from build123d import *

# Parameters (mm, degrees)
SKETCH1_W           = 17.4
SKETCH1_H           = 16.3
BOSS_EXTRUDE1_DEPTH = 5.6
SKETCH2_R           = 4.25
BOSS_EXTRUDE2_DEPTH = 7
SKETCH3_R           = 2.9
BOSS_EXTRUDE3_DEPTH = 13
FILLET1_R           = 3
SKETCH4_W           = 3.8
SKETCH4_H           = 0.8
BOSS_EXTRUDE4_DEPTH = 2.9
FILLET2_R           = 1
BOSS_EXTRUDE5_DEPTH = 2.3


with BuildPart() as part:
    # Sketch1 → Boss-Extrude1 (new body)
    with BuildSketch(Plane(origin=(0, 0, 0), x_dir=(1, 0, 0), z_dir=(0, 1, 0))):
        Rectangle(SKETCH1_W, SKETCH1_H)
    extrude(amount=BOSS_EXTRUDE1_DEPTH)

    # Sketch2 → Boss-Extrude2 (add)
    with BuildSketch(Plane(origin=(0, 5.6, 0), x_dir=(1, 0, 0), z_dir=(0, 1, 0))):
        with Locations(Location((0, 0, 0), (0, 0, 270))):  # turned: the seam where the file's is
            Circle(SKETCH2_R)
    extrude(amount=BOSS_EXTRUDE2_DEPTH)

    # Sketch3 → Boss-Extrude3 (add)
    with BuildSketch(Plane(origin=(0, 12.6, 0), x_dir=(1, 0, 0), z_dir=(0, 1, 0))):
        with Locations(Location((0, 0, 0), (0, 0, 270))):  # turned: the seam where the file's is
            Circle(SKETCH3_R)
    extrude(amount=BOSS_EXTRUDE3_DEPTH)

    # Fillet1
    fillet1_edges = [part.edges().sort_by_distance(p)[0] for p in [
        (-8.7, 2.8, -8.15),
        (-8.7, 2.8, 8.15),
    ]]
    fillet(fillet1_edges, radius=FILLET1_R)

    # Sketch4 → Boss-Extrude4 (add)
    with BuildSketch(Plane(origin=(8.7, 0, 0), x_dir=(0, 0, -1), z_dir=(1, 0, 0))):
        with Locations((0, 5.2)):
            Rectangle(SKETCH4_W, SKETCH4_H)
    extrude(amount=BOSS_EXTRUDE4_DEPTH)

    # Fillet2
    fillet2_edges = [part.edges().sort_by_distance(p)[0] for p in [
        (8.7, 5.2, -1.9),
        (8.7, 5.2, 1.9),
    ]]
    fillet(fillet2_edges, radius=FILLET2_R)

    # Sketch5 → Boss-Extrude5 (add)
    with BuildSketch(Plane(origin=(0, 5.6, 0), x_dir=(1, 0, 0), z_dir=(0, 1, 0))):
        with BuildLine():
            Line((8.7, 1.4), (8.7, -1.4))
            ThreePointArc((8.7, -1.4), (10.1, 0), (8.7, 1.4))
        make_face()
    extrude(amount=BOSS_EXTRUDE5_DEPTH)


solid = part.part
Read the model definition and answer for the solid it produces. Units are mm, in the model's axes. A direction names the side the tool comes from. Coordinates: 2 decimals unless noted, no trailing zeros. Order: outer loops, then holes, each group sorted by start corner. A loop starts at its lowest first (then second) coordinate and runs counter-clockwise, first axis right, second up. Notation, with made-up numbers: M 64.5,51.25 L 112.5,51.25 A9 cw 112.5,57.25 Z; hole C -15,-23.75 d7. An arc over 180 degrees is marked long. Put each result on its own line as item: value. Start each with the question number.
Item 1: For faces 4 (the face through (9, 7.9, 0)), 5 (the face through (10, 4.8, 0)), 6 (the face through (10.1, 6.7, 0)), determine the directions among +Z, -Z, +X, -X, +Y, -Y from which every point of the face is accessible in a straight line to the end or side of a thin tool.
Item 2: Given pin 1 Ø1.7 at (y, z) = (3, 2) entering from +X; pin 2 Ø0.7 at (y, z) = (7.5, 0.5) entering from -X; pin 3 Ø1 at (y, z) = (16, -0.5) entering from +X; pin 4 Ø3 at (x, z) = (2, 2) entering from -Y, each flat-ended and moving along its own axis, determine where each tip first touches the part or whether it passes through.
Item 3: Section B-B, the plane x = 0 is taken. Determine the outline of the cut face in (y, z).
Item 4: The mould has two halves that part along X. Classify faces 1 (the face through (8.7, 7, 0)), 2 (the face through (0.1, 19, -2.9)), 3 (the face through (-3, 12.6, 1)): +X half, -X half, draft (parallel to the pull), parting line (faces both ways), or undercut.
Item 5: Section D-D, the plane z = 0 is taken. Determine the outline of the cut face in (x, y).
Item 6: Section A-A, the plane z = -3.75 is taken. Determine the outline of the cut face in (x, y), plus the area to 3 significant figures.
Item 7: Consider probe 1 along Y at (x, z) = (7.25, 6.75); probe 2 along Y at (x, z) = (-2.25, 2); probe 3 along X at (y, z) = (3.5, -4.5). Determine where each line is inside the solid, lowest interval first. Write a range as [from, to].
Item 8: Section C-C, the plane y = 18.5 is taken. Determine the outline of the cut face in (x, z), plus the area to 3 significant figures.
Computed:
1. face 4: +Z, -Z, +X, +Y
1. face 5: +Z, -Z, +X, -Y
1. face 6: +X, +Y
2. pin 1: stops at x = 8.7
2. pin 2: stops at x = -4.25
2. pin 3: stops at x = 2.9
2. pin 4: stops at y = 0
3. outline: M 0,-8.15 L 5.6,-8.15 L 5.6,-4.25 L 12.6,-4.25 L 12.6,-2.9 L 25.6,-2.9 L 25.6,2.9 L 12.6,2.9 L 12.6,4.25 L 5.6,4.25 L 5.6,8.15 L 0,8.15 Z
4. face 1: undercut
4. face 2: parting line
4. face 3: draft
5. outline: M -8.7,0 L 8.7,0 L 8.7,4.8 L 11.6,4.8 L 11.6,5.6 L 10.1,5.6 L 10.1,7.9 L 8.7,7.9 L 8.7,5.6 L 4.25,5.6 L 4.25,12.6 L 2.9,12.6 L 2.9,25.6 L -2.9,25.6 L -2.9,12.6 L -4.25,12.6 L -4.25,5.6 L -8.7,5.6 Z
6. outline: M -8.7,0 L 8.7,0 L 8.7,5.6 L 2,5.6 L 2,12.6 L -2,12.6 L -2,5.6 L -8.7,5.6 Z
6. area: 125 mm2
7. probe 1: y = [0, 5.6]
7. probe 2: y = [0, 12.6]
7. probe 3: x = [-8.7, 8.7]
8. outline: C 0,0 d5.8
8. area: 26.4 mm2
